Geometry check sheet. Reference: drawing and pictorial views, mm from the part's lowest x, y, z. A direction names the side the tool comes from. Coordinates: 2 decimals unless noted, no trailing zeros. Order: outer loops, then holes, each group sorted by start corner. A loop starts at its lowest first (then second) coordinate and runs counter-clockwise, first axis right, second up. Notation, with made-up numbers: M 56,39.5 L 84,39.5 A28 cw 84,69.5 Z; hole C -25,53 d6. An arc over 180 degrees is marked long. Return JSON: item names as keys, results as strings.
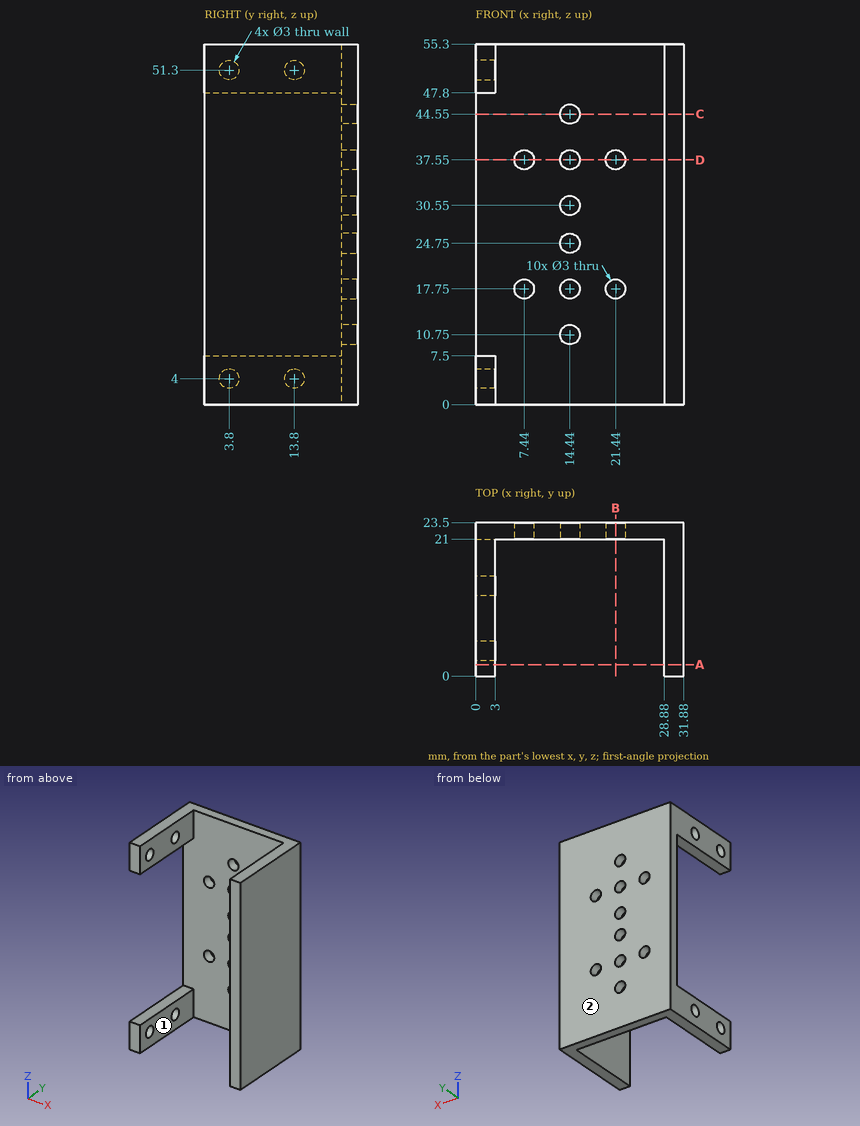
Q1. Cross-section at D-D, the plane z = 37.55. Record the boundary of the cut face in (x, y).
Values:
{"outline": "M 0,21 L 5.94,21 L 5.94,23.5 L 0,23.5 Z; M 8.94,21 L 12.94,21 L 12.94,23.5 L 8.94,23.5 Z; M 15.94,21 L 19.94,21 L 19.94,23.5 L 15.94,23.5 Z; M 22.94,21 L 28.88,21 L 28.88,0 L 31.88,0 L 31.88,23.5 L 22.94,23.5 Z"}
Q2. Cross-section at B-B, the plane x = 21.44. Record the boundary of the cut face in (y, z), and give its area (3 significant figures).
Values:
{"outline": "M 21,0 L 23.5,0 L 23.5,16.25 L 21,16.25 Z; M 21,19.25 L 23.5,19.25 L 23.5,36.05 L 21,36.05 Z; M 21,39.05 L 23.5,39.05 L 23.5,55.3 L 21,55.3 Z", "area": "123 mm^2"}
Q3. Go/stop test with flat-tipped pins: pin 1 (3.5 mm diameter, centred on x = 14.44, z = 10.75, fed in from -Y); pin 2 (2.5 mm diameter, centred on y = 3.8, z = 51.3, fed in from -X). Record where each tip stops, or that it passes through.
Values:
{"pin 1": "y = 21", "pin 2": "x = 28.88"}
Q4. Material ranges on line 1 along X through (y, z) = (21.9, 17.75); line 2 along Y through (x, z) = (1.65, 51.3); line 3 along X through (y, z) = (22.9, 10.75), recorded low to high.
Values:
{"line 1": "0 to 5.94, 8.94 to 12.94, 15.94 to 19.94, 22.94 to 31.88", "line 2": "0 to 2.3, 5.3 to 12.3, 15.3 to 23.5", "line 3": "0 to 12.94, 15.94 to 31.88"}
Q5. Cross-section at C-C, the plane z = 44.55. Record the boundary of the cut face in (x, y).
Values:
{"outline": "M 0,21 L 12.94,21 L 12.94,23.5 L 0,23.5 Z; M 15.94,21 L 28.88,21 L 28.88,0 L 31.88,0 L 31.88,23.5 L 15.94,23.5 Z"}
Q6. Cross-section at A-A, the plane y = 1.75. Record the boundary of the cut face in (x, z).
Values:
{"outline": "M 0,0 L 3,0 L 3,7.5 L 0,7.5 Z; M 0,47.8 L 3,47.8 L 3,55.3 L 0,55.3 Z; M 28.88,0 L 31.88,0 L 31.88,55.3 L 28.88,55.3 Z"}
Q7. Tool access check on the marked faces 1 and 2. Record the directions out of +Z, -Z, +X, -X, +Y, -Y that give a thin tool (end or side, any length) a straight path to the whole face; none if there is none.
Values:
{"face 1": "+Z, -Z, -Y", "face 2": "+Z, -Z, +X, -X, +Y"}
